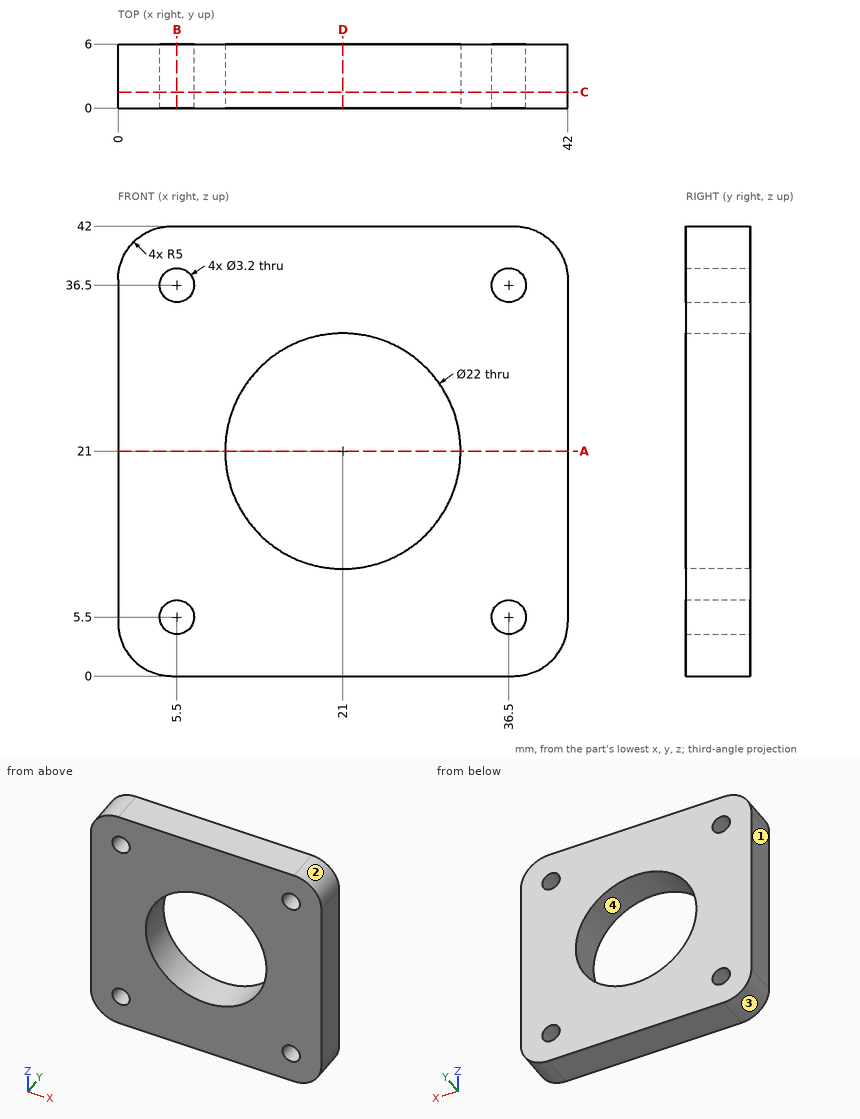
Design review of the part shown in the three views and the two pictorial views. Dimensions are in mm from the part's minimum x, y and z. Coordinates: 2 decimals unless noted, no trailing zeros. Loops run counter-clockwise (first coordinate to the right, second up) from the corner with the lowest first, then second, coordinate; pieces in that order, holes last. Notation, with made-up numbers: (-5, 28) -> (24, 28) arc R14 cw to (24, 41) -> close; hole circle Ø9 at (67, 89). An arc over 180 degrees is marked (long way). Answer as CSV lines item,"result".
Item 1: Take a section at A-A, the plane z = 21. State the section outline as (x, y) points.
Results below:
outline,"(0, 0) -> (10, 0) -> (10, 6) -> (0, 6) -> close; (32, 0) -> (42, 0) -> (42, 6) -> (32, 6) -> close"
Item 2: Insertion check: pin 1 (4 mm diameter, centred on x = 5.5, z = 36.5, fed in from +Y). The pin has a flat end and moves straight along its axis. Give the tip position at first contact, or say it passes through.
Results below:
pin 1,"stops at y = 6"
Item 3: Draft analysis for pull direction Z (two halves, no side actions). For the marked faces 1, 2, 3 and 4, state which applies: +Z half, -Z half, draft (parallel to the pull), parting line (faces both ways), or undercut.
Results below:
face 1,"draft"
face 2,"+Z half"
face 3,"-Z half"
face 4,"undercut"
Item 4: Take a section at B-B, the plane x = 5.5. State the section outline as (y, z) points.
Results below:
outline,"(0, 0) -> (6, 0) -> (6, 3.9) -> (0, 3.9) -> close; (0, 7.1) -> (6, 7.1) -> (6, 34.9) -> (0, 34.9) -> close; (0, 38.1) -> (6, 38.1) -> (6, 42) -> (0, 42) -> close"
Item 5: For L1, parallel to X at y = 2.5, z = 36.5; L2, parallel to X at y = 0.5, z = 37; L3, parallel to X at y = 4, z = 21, list the stretches that pass through material, from the lowest coordinate up.
Results below:
L1,"x = 0 to 3.9, 7.1 to 34.9, 38.1 to 42"
L2,"x = 0 to 3.98, 7.02 to 34.98, 38.02 to 42"
L3,"x = 0 to 10, 32 to 42"
Item 6: Take a section at C-C, the plane y = 1.5. State the section outline as (x, z) points.
Results below:
outline,"(0, 5) arc R5 ccw to (5, 0) -> (37, 0) arc R5 ccw to (42, 5) -> (42, 37) arc R5 ccw to (37, 42) -> (5, 42) arc R5 ccw to (0, 37) -> close; hole circle Ø3.2 at (5.5, 5.5); hole circle Ø3.2 at (5.5, 36.5); hole circle Ø22 at (21, 21); hole circle Ø3.2 at (36.5, 5.5); hole circle Ø3.2 at (36.5, 36.5)"
Item 7: Take a section at D-D, the plane x = 21. State the section outline as (y, z) points.
Results below:
outline,"(0, 0) -> (6, 0) -> (6, 10) -> (0, 10) -> close; (0, 32) -> (6, 32) -> (6, 42) -> (0, 42) -> close"
